Model file for the job. Use its own axes, mm. Face numbers are marked on the shaded views. Give positions to 0.01 mm unless a question says otherwise; leave off trailing zeros. Order: outer loops, then holes, each group sorted by start corner. A loop starts at its lowest first (then second) coordinate and runs counter-clockwise, first axis right, second up. Notation, with made-up numbers: (-7.5, -33) -> (23.5, -33) arc R23 cw to (23.5, -24) -> close; hole circle Ø10 at (-19.5, 8). An arc over 180 degrees is marked (long way). Answer in a Markdown table with one row per item. Add a question column.
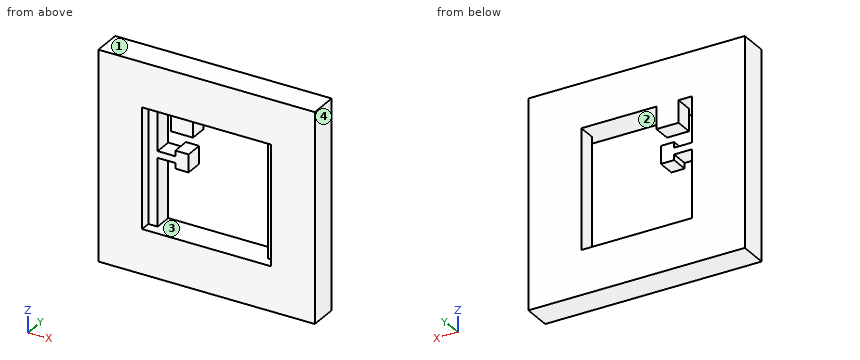
from build123d import *

# Parameters (mm, degrees)
SKETCH1_W           = 49
SKETCH1_H           = 47
BOSS_EXTRUDE1_DEPTH = 4
SKETCH2_W           = 49
SKETCH2_H           = 47
SKETCH2_W_2         = 29.2
SKETCH2_H_2         = 27
BOSS_EXTRUDE2_DEPTH = 2.4


with BuildPart() as part:
    # Sketch1 → Boss-Extrude1 (new body)
    with BuildSketch(Plane(origin=(0, 0, 0), x_dir=(1, 0, 0), z_dir=(0, 1, 0))):
        Rectangle(SKETCH1_W, SKETCH1_H)
        Polygon((-12.5, -13.5), (-9.5, -13.5), (-9.5, -8.5), (-4.5, -8.5), (-4.5, -13.5), (12.5, -13.5), (12.5, 13.5), (-12.5, 13.5), (-12.5, -1.75), (-8.5, -1.75), (-8.5, -0.5), (-5.5, -0.5), (-5.5, -4.5), (-8.5, -4.5), (-8.5, -3.25), (-12.5, -3.25), align=None, mode=Mode.SUBTRACT)
    extrude(amount=BOSS_EXTRUDE1_DEPTH)

    # Sketch2 → Boss-Extrude2 (add)
    with BuildSketch(Plane.XZ):
        Rectangle(SKETCH2_W, SKETCH2_H)
        Rectangle(SKETCH2_W_2, SKETCH2_H_2, mode=Mode.SUBTRACT)
    extrude(amount=BOSS_EXTRUDE2_DEPTH)


solid = part.part
Item 1: Wall check: line 1 (Z direction, x = -10, y = 2.25); line 2 (Z direction, x = -9, y = 0.75); line 3 (X direction, y = 1.75, z = 0). Give the ranges that are in metal, low to high.
Item 2: Two-plate mould, pull along Z, no slides. Class the marked faces 1, 2, 3 and 4: pulls with the +Z half, pulls with the -Z half, needs draft (parallel to the pull), parting line crosses it, or undercut.
Item 3: Saw through at C-C on x = 5.5. List the corners of the cut face in (y, z), plus the area to 3 significant figures.
Item 4: Saw through at A-A on y = -1. List the corners of the cut face in (x, z), plus the area to 3 significant figures.
Item 5: Pin check, flat tip, straight feed: pin 1 Ø2 at (x, z) = (13.5, -1.5) entering from -Y. Stop position of the tip, or through.
Item 6: Saw through at B-B on z = 7. List the corners of the cut face in (x, y).
Evaluation:
| question | item | result |
|---|---|---|
| 1 | line 1 | z = -23.5 to -13.5, 1.75 to 3.25, 13.5 to 23.5 |
| 1 | line 2 | z = -23.5 to -13.5, 1.75 to 3.25, 8.5 to 23.5 |
| 1 | line 3 | x = -24.5 to -12.5, 12.5 to 24.5 |
| 2 | face 1 | pulls with the +Z half |
| 2 | face 2 | undercut |
| 2 | face 3 | undercut |
| 2 | face 4 | needs draft |
| 3 | outline | (-2.4, -23.5) -> (4, -23.5) -> (4, -13.5) -> (-2.4, -13.5) -> close; (-2.4, 13.5) -> (4, 13.5) -> (4, 23.5) -> (-2.4, 23.5) -> close |
| 3 | area | 128 mm2 |
| 4 | outline | (-24.5, -23.5) -> (24.5, -23.5) -> (24.5, 23.5) -> (-24.5, 23.5) -> close; hole (-14.6, -13.5) -> (14.6, -13.5) -> (14.6, 13.5) -> (-14.6, 13.5) -> close |
| 4 | area | 1,510 mm2 |
| 5 | pin 1 | stops at y = 0 |
| 6 | outline | (-24.5, -2.4) -> (-14.6, -2.4) -> (-14.6, 0) -> (-12.5, 0) -> (-12.5, 4) -> (-24.5, 4) -> close; (12.5, 0) -> (14.6, 0) -> (14.6, -2.4) -> (24.5, -2.4) -> (24.5, 4) -> (12.5, 4) -> close |
